Geometry: see drawing. Coordinates: mm, zero at the bounding-box minimum. A direction names the side the tool comes from. Coordinates: 2 decimals unless noted, no trailing zeros. Loops run counter-clockwise (first coordinate to the right, second up) from the corner with the lowest first, then second, coordinate; pieces in that order, holes last. Notation, with made-up numbers: (69.25, -28) - (83.25, -28) arc R19 cw to (83.25, -18) - close; hole circle Ø2 at (24, -27). An arc over 180 degrees is marked (long way). Use a Markdown table: item, result. Add a question column.
1. Section query D-D on y = 56. Return the cut outline in (x, z), then the cut area to 3 significant figures.
2. Contact query for flat-ended pins moving along their axis: P1, Ø6, axis at x = 25.5, z = 45.5, coming from the +Y side; P2, Ø12, axis at x = 18, z = 43, coming from the -Y side; P3, Ø6, axis at x = 8, y = 8.5, coming from the -Z side. Output: stop coordinate, or through.
3. Section query A-A on x = 19.5. Return the cut outline in (y, z), then the cut area to 3 significant figures.
4. Draft query along Z for the marked faces 1, 2 and 3. Return one class per face: released by +Z, released by -Z, zero draft, split by the parting line, or undercut.
5. Section query C-C on x = 38. Return the cut outline in (y, z).
6. Access query for the marked faces 4, 5, 6 and 7. Directions: +Z, -Z, +X, -X, +Y, -Y. A direction counts if a zero-diameter tool reaches every point of the face in a straight line with its end or side. Return the directions, or none.
7. Section query B-B on z = 19.5. Return the cut outline in (x, y), then the cut area to 3 significant figures.
8. Ray query, L1, parallel to Z at x = 23.5, y = 37.7; L2, parallel to Y at x = 14.5, z = 30; L3, parallel to Z at x = 5, y = 36.5. Return the intervals inside material, ascending. Write a range as [from, to].
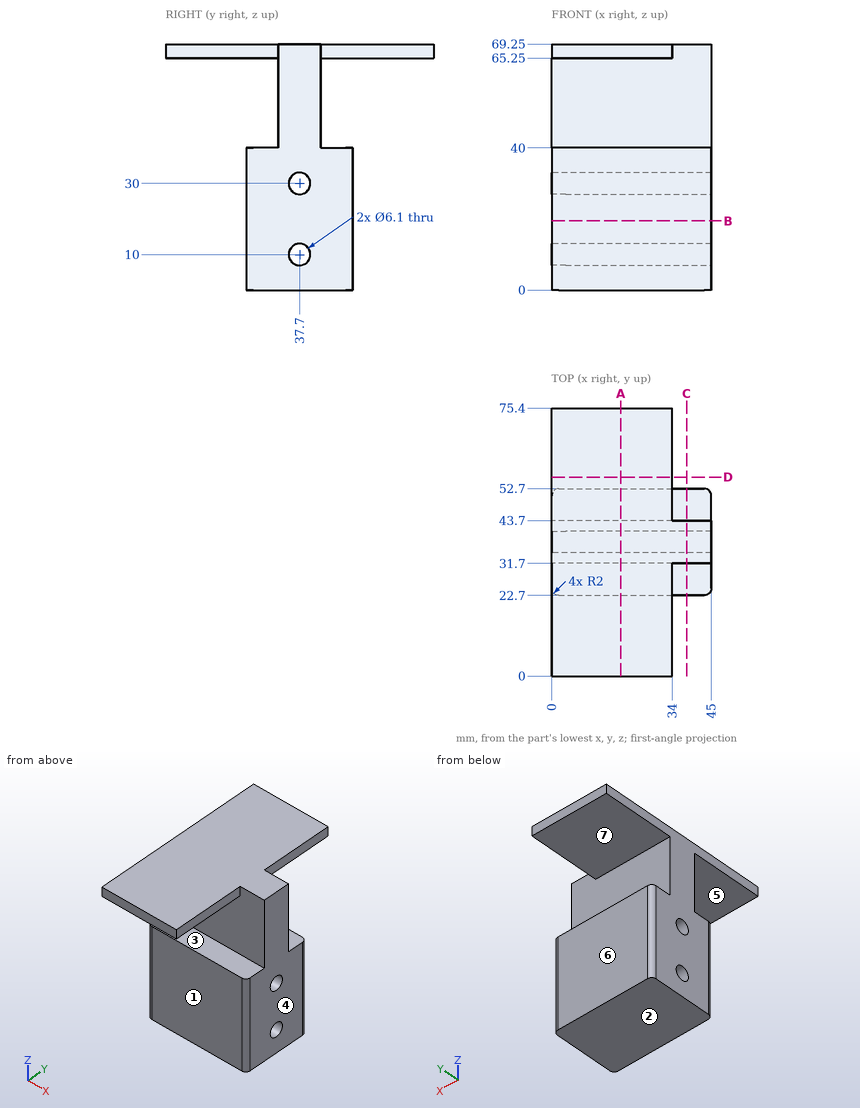
Resolved:
| question | item | result |
|---|---|---|
| 1 | outline | (0, 65.25) - (34, 65.25) - (34, 69.25) - (0, 69.25) - close |
| 1 | area | 136 mm² |
| 2 | P1 | y = 43.7 |
| 2 | P2 | y = 22.7 |
| 2 | P3 | z = 65.25 |
| 3 | outline | (0, 65.25) - (31.7, 65.25) - (31.7, 40) - (22.7, 40) - (22.7, 0) - (52.7, 0) - (52.7, 40) - (43.7, 40) - (43.7, 65.25) - (75.4, 65.25) - (75.4, 69.25) - (0, 69.25) - close; hole circle Ø6.1 at (37.7, 10); hole circle Ø6.1 at (37.7, 30) |
| 3 | area | 1,750 mm² |
| 4 | face 1 | zero draft |
| 4 | face 2 | released by -Z |
| 4 | face 3 | undercut |
| 5 | outline | (22.7, 0) - (52.7, 0) - (52.7, 40) - (43.7, 40) - (43.7, 69.25) - (31.7, 69.25) - (31.7, 40) - (22.7, 40) - close; hole circle Ø6.1 at (37.7, 10); hole circle Ø6.1 at (37.7, 30) |
| 6 | face 4 | +Z, -Z, +X, +Y, -Y |
| 6 | face 5 | +X, -X, -Y |
| 6 | face 6 | -Z, +X, -X, +Y |
| 6 | face 7 | +X, -X, +Y |
| 7 | outline | (0, 24.7) arc R2 ccw to (2, 22.7) - (43, 22.7) arc R2 ccw to (45, 24.7) - (45, 50.7) arc R2 ccw to (43, 52.7) - (2, 52.7) arc R2 ccw to (0, 50.7) - close |
| 7 | area | 1,350 mm² |
| 8 | L1 | [0, 6.95], [13.05, 26.95], [33.05, 69.25] |
| 8 | L2 | [22.7, 34.65], [40.75, 52.7] |
| 8 | L3 | [0, 7.2], [12.8, 27.2], [32.8, 69.25] |
